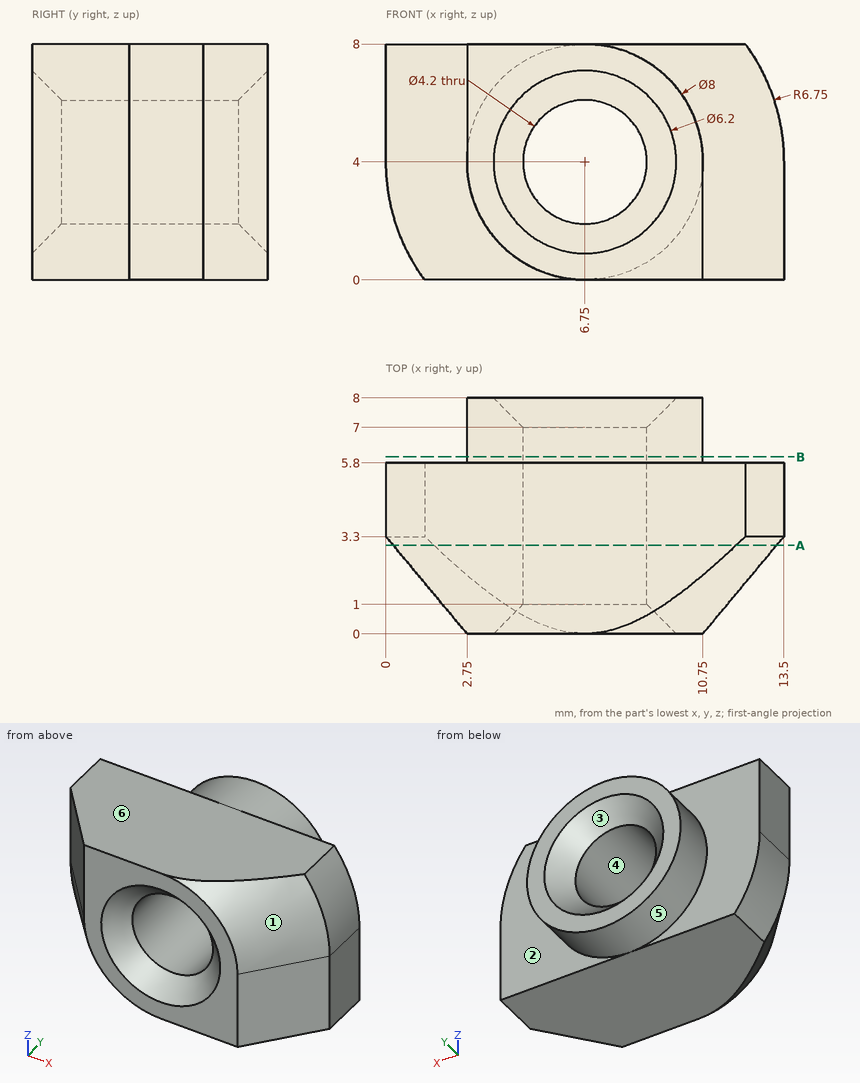
The figure shows three views and two pictorial views of one solid part (mm, origin at its lowest corner). Answer the questions. A direction names the side the tool comes from. Coordinates: 2 decimals unless noted, no trailing zeros. Loops run counter-clockwise (first coordinate to the right, second up) from the corner with the lowest first, then second, coordinate; pieces in that order, holes last.
1) Find the intervals of material crossed by L1, parallel to Y at x = 10.25, z = 1.5; L2, parallel to Z at x = 7.75, y = 1.25; L3, parallel to X at y = 2.25, z = 3 (3 decimals), in increasing order.
2) Find section B-B on y = 6. Write down the section's boundary in (x, z).
3) A tool of negligible diameter and unlimited length cuts with its end or side. For the marked faces 5 and 6, from which of +Z, -Z, +X, -X, +Y, -Y can it reach the whole face along a straight path? Write none if from no direction.
4) Find section A-A on y = 3. Write down the section's boundary in (x, z), then the cut area to 3 significant figures.
5) Determine the mould class of the marked faces 1, 2, 3 and 4 for opening direction X: pulls with the +X half, pulls with the -X half, needs draft (parallel to the pull), parting line crosses it, or undercut.
6) Flat-ended cylindrical pins translate along their axes: pin 1 Ø1 at (y, z) = (2.5, 3) entering from +X; pin 2 Ø2 at (x, z) = (8.5, 5) entering from +Y. Find the tip coordinate at first contact, or state that the pin passes through.
Values:
1. L1: y = 0 to 5.8
1. L2: z = 0 to 2.15, 5.85 to 8
1. L3: x = 0.961 to 4.903, 8.597 to 12.625
2. outline: circle Ø8 at (6.75, 4); hole circle Ø4.2 at (6.75, 4)
3. face 5: +Y
3. face 6: +Z, +X, -X, +Y, -Y
4. outline: (0.25, 4) arc R6.5 ccw to (1.63, 0) - (13.25, 0) - (13.25, 4) arc R6.5 ccw to (11.87, 8) - (0.25, 8) - close; hole circle Ø4.2 at (6.75, 4)
4. area: 86.6 mm2
5. face 1: pulls with the +X half
5. face 2: needs draft
5. face 3: undercut
5. face 4: undercut
6. pin 1: stops at x = 13.25
6. pin 2: stops at y = 7.92
